Source: CAD feature listing. Evaluate the final solid. Frame: model axes, mm. Coordinates: 2 decimals unless noted, no trailing zeros. Write each loop counter-clockwise with the first axis right and the second up, starting at its lowest first coordinate (ties: lowest second). Pieces come first, ordered by that corner, then holes. Notation, with made-up numbers: (27.5, 49) - (45.5, 49) arc R10 cw to (45.5, 64) - close; hole circle Ø10 at (-32, -26.5). An arc over 180 degrees is marked (long way). One line per question, with ' | ' between items.
from build123d import *

# Parameters (mm, degrees)
SKETCH1_R           = 2.54
SKETCH1_W           = 12.7
SKETCH1_H           = 38.1
BOSS_EXTRUDE1_DEPTH = 3.175
SKETCH4_R           = 2.54
CUT_EXTRUDE2_DEPTH  = 25.4


with BuildPart() as part:
    # Sketch1 → Boss-Extrude1 (new body)
    # profile 1 of 3: a face of its own
    with BuildSketch(Plane(origin=(0, 0, 0), x_dir=(1, 0, 0), z_dir=(0, 1, 0))):
        Polygon((0.840595698, 5.08), (19.05, 5.08), (37.259404302, 5.08), (30.48, 46.0502), (7.62, 46.0502), align=None)
        with Locations(Location((8.509, 10.3124, 0), (0, 0, 270))):
            Circle(SKETCH1_R, mode=Mode.SUBTRACT)
        with Locations(Location((29.591, 10.3124, 0), (0, 0, 270))):
            Circle(SKETCH1_R, mode=Mode.SUBTRACT)
        with Locations(Location((19.05, 36.9316, 0), (0, 0, 270))):
            Circle(SKETCH1_R, mode=Mode.SUBTRACT)
    # profile 2 of 3: a face of its own
    with BuildSketch(Plane(origin=(0, 0, 0), x_dir=(1, 0, 0), z_dir=(0, 1, 0))):
        Polygon((12.7, 76.750333333), (7.62, 46.0502), (30.48, 46.0502), (25.4, 76.750333333), align=None)
    # profile 3 of 3: a face of its own
    with BuildSketch(Plane(origin=(0, 0, 0), x_dir=(1, 0, 0), z_dir=(0, 1, 0))):
        with Locations((19.05, 95.800333333)):
            Rectangle(SKETCH1_W, SKETCH1_H)
    extrude(amount=BOSS_EXTRUDE1_DEPTH)

    # Sketch4 → Cut-Extrude2 (cut)
    with BuildSketch(Plane.XZ):
        with Locations(Location((19.05, -72.39, 0), (0, 0, 270))):
            Circle(SKETCH4_R)
        with Locations(Location((19.05, -89.450333333, 0), (0, 0, 270))):
            Circle(SKETCH4_R)
    extrude(amount=-CUT_EXTRUDE2_DEPTH, mode=Mode.SUBTRACT)


solid = part.part
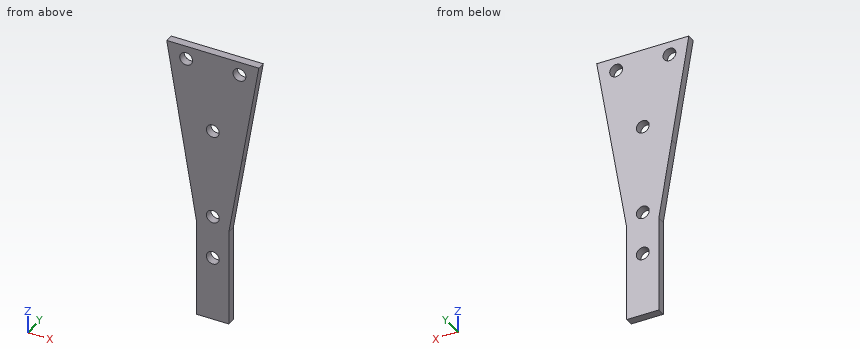
Item 1: Cut plane A-A on x = 19.05. Return loops of the section in (y, z) (3 decimals).
Check sheet entries:
outline: (0, -114.85) - (3.175, -114.85) - (3.175, -91.99) - (0, -91.99) - close; (0, -86.91) - (3.175, -86.91) - (3.175, -74.93) - (0, -74.93) - close; (0, -69.85) - (3.175, -69.85) - (3.175, -39.472) - (0, -39.472) - close; (0, -34.392) - (3.175, -34.392) - (3.175, -5.08) - (0, -5.08) - close
Item 2: Cut plane B-B on z = -72.39. Return loops of the section in (x, y) (3 decimals), and give its area (3 significant figures).
Check sheet entries:
outline: (11.978, 0) - (16.51, 0) - (16.51, 3.175) - (11.978, 3.175) - close; (21.59, 0) - (26.122, 0) - (26.122, 3.175) - (21.59, 3.175) - close | area: 28.8 mm²
Item 3: Cut plane D-D on z = -103. Return loops of the section in (x, y) (3 decimals), and give its area (3 significant figures).
Check sheet entries:
outline: (12.7, 0) - (25.4, 0) - (25.4, 3.175) - (12.7, 3.175) - close | area: 40.3 mm²
Item 4: Ray query, line 1 along X through (y, z) = (2.05, -84); line 2 along X through (y, z) = (1.95, -24); line 3 along X through (y, z) = (2.05, -37.5). Return the intervals inside material, ascending. Write a range as [from, to].
Check sheet entries:
line 1: [12.7, 25.4] | line 2: [3.97, 34.13] | line 3: [6.21, 16.57], [21.53, 31.89]
Item 5: Pin query (flat end, axial travel): pin 1 Ø3 at (x, z) = (28.5, -39.5) entering from -Y; pin 2 Ø1 at (y, z) = (2, -100) entering from -X. Return the tip coordinate at first contact, or that it passes through.
Check sheet entries:
pin 1: y = 0 | pin 2: x = 12.7
Item 6: Cut plane C-C on y = 2.6. Return loops of the section in (x, z), and give its area (3 significant figures).
Check sheet entries:
outline: (0.84, -5.08) - (12.7, -76.75) - (12.7, -114.85) - (25.4, -114.85) - (25.4, -76.75) - (37.26, -5.08) - close; hole circle Ø5.08 at (8.51, -10.31); hole circle Ø5.08 at (19.05, -89.45); hole circle Ø5.08 at (19.05, -72.39); hole circle Ø5.08 at (19.05, -36.93); hole circle Ø5.08 at (29.59, -10.31) | area: 2,140 mm²
